from build123d import *

# Parameters (mm, degrees)
F0_W     = 101.6
F0_H     = 127
F1_DEPTH = 19.05
F2_W     = 76.2
F2_H     = 19.05
F3_DEPTH = 9.525
F4_R     = 6.35
F6_DEPTH = 19.051
F7_R     = 5.08
F8_W     = 25.4
F8_H     = 19.05
F9_DEPTH = 127.001


with BuildPart() as f1:
    # F0 (on Top) → F1 (new body)
    with BuildSketch(Plane.XY):
        with Locations((50.8, 63.5)):
            Rectangle(F0_W, F0_H)
    extrude(amount=F1_DEPTH)

    # F2 (on face) → F3 (cut)
    with BuildSketch(Plane.XY.offset(19.05)):
        with Locations((38.1, 63.5)):
            Rectangle(F2_W, F2_H)
    extrude(amount=-F3_DEPTH, mode=Mode.SUBTRACT)

    # F4
    f4_edges = [f1.edges().sort_by_distance(p)[0] for p in [
        (76.2, 73.025, 14.2875),
        (76.2, 53.975, 14.2875),
    ]]
    fillet(f4_edges, radius=F4_R)

    # F5 (on face) → F6 (cut, through all)
    with BuildSketch(Plane.XY.offset(19.05)):
        with BuildLine():
            ThreePointArc((25.4, 34.925), (22.225, 31.75), (25.4, 28.575))
            Line((25.4, 28.575), (76.2, 28.575))
            ThreePointArc((76.2, 28.575), (79.375, 31.75), (76.2, 34.925))
            Line((76.2, 34.925), (25.4, 34.925))
        make_face()
        with BuildLine():
            ThreePointArc((25.4, 98.425), (22.225, 95.25), (25.4, 92.075))
            Line((25.4, 92.075), (76.2, 92.075))
            ThreePointArc((76.2, 92.075), (79.375, 95.25), (76.2, 98.425))
            Line((76.2, 98.425), (25.4, 98.425))
        make_face()
    extrude(amount=-F6_DEPTH, mode=Mode.SUBTRACT)

    # F7
    f7_edges = [f1.edges().sort_by_distance(p)[0] for p in [
        (101.6, 0, 9.525),
        (101.6, 127, 9.525),
    ]]
    fillet(f7_edges, radius=F7_R)

    # F8 (on face) → F9 (cut, through all)
    with BuildSketch(Plane.XZ):
        with Locations((-3.175, 19.05)):
            Rectangle(F8_W, F8_H)
    extrude(amount=-F9_DEPTH, mode=Mode.SUBTRACT)


solid = f1.part
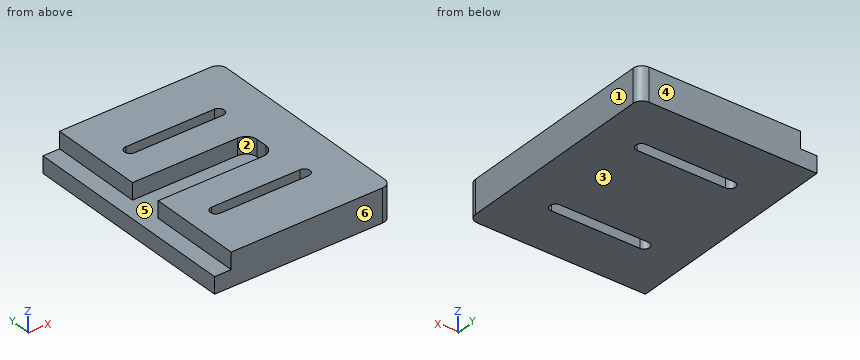
Verification items for the finished model (mm, model axes). Face numbers are marked on the shaded views. A direction names the side the tool comes from. Round coordinates to 2 decimals unless told otherwise and drop trailing zeros. Loops run counter-clockwise (first coordinate to the right, second up) from the corner with the lowest first, then second, coordinate; pieces in that order, holes last. Notation, with made-up numbers: M -26.5,63.25 L 13.5,63.25 A11 ccw 13.5,70.25 Z; hole C -5.75,0 d8. An arc over 180 degrees is marked long. Write each question's results on one line, items separated by ' | '.
1) Section check D-D on x = 15. Record the boundary of the cut face in (y, z) (3 decimals).
Checks:
outline: M 0,0 L 127,0 L 127,19.05 L 73.025,19.05 L 73.025,9.525 L 53.975,9.525 L 53.975,19.05 L 0,19.05 Z
2) Section check C-C on z = 16. Record the boundary of the cut face in (x, y) (3 decimals), then the cut area to 3 significant figures.
Checks:
outline: M 9.525,0 L 96.52,0 A5.08 ccw 101.6,5.08 L 101.6,121.92 A5.08 ccw 96.52,127 L 9.525,127 L 9.525,73.025 L 69.85,73.025 A6.35 cw 76.2,66.675 L 76.2,60.325 A6.35 cw 69.85,53.975 L 9.525,53.975 Z; hole M 25.4,28.575 L 76.2,28.575 A3.175 ccw 76.2,34.925 L 25.4,34.925 A3.175 ccw Z; hole M 25.4,92.075 L 76.2,92.075 A3.175 ccw 76.2,98.425 L 25.4,98.425 A3.175 ccw Z | area: 9,720 mm2
3) Section check B-B on x = 59. Record the boundary of the cut face in (y, z) (3 decimals).
Checks:
outline: M 0,0 L 28.575,0 L 28.575,19.05 L 0,19.05 Z; M 34.925,0 L 92.075,0 L 92.075,19.05 L 73.025,19.05 L 73.025,9.525 L 53.975,9.525 L 53.975,19.05 L 34.925,19.05 Z; M 98.425,0 L 127,0 L 127,19.05 L 98.425,19.05 Z
4) Section check A-A on y = 95.25. Record the boundary of the cut face in (x, z) (3 decimals).
Checks:
outline: M 0,0 L 22.225,0 L 22.225,19.05 L 9.525,19.05 L 9.525,9.525 L 0,9.525 Z; M 79.375,0 L 101.6,0 L 101.6,19.05 L 79.375,19.05 Z
5) Access from +Z, -Z, +X, -X, +Y, -Y to the whole of each face (thin tool, end or side, straight path). Record for the marked faces 1 and 2.
Checks:
face 1: +Z, -Z, +X, +Y, -Y | face 2: +Z, -X
6) Gauge pin test, flat ends, axial feed: P1, Ø3, axis at y = 63.5, z = 16, coming from the -X side; P2, Ø3, axis at y = 99, z = 12.5, coming from the -X side (3 decimals). Record the tip position at first contact, or that the pin passes through.
Checks:
P1: stops at x = 76.2 | P2: stops at x = 9.525
7) Scan lines: L1, parallel to Y at x = 33.5, z = 14.5 (3 decimals); L2, parallel to Y at x = 29, z = 1.25 (3 decimals); L3, parallel to Y at x = 24, z = 17.5 (3 decimals). Record each from-to range of solid material in increasing order. Write a range as from..to.
Checks:
L1: y = 0..28.575, 34.925..53.975, 73.025..92.075, 98.425..127 | L2: y = 0..28.575, 34.925..92.075, 98.425..127 | L3: y = 0..28.9, 34.6..53.975, 73.025..92.4, 98.1..127
8) Mould release check, pull along Y, two halves, no side actions. Record for the marked faces 3, 4, 5 and 6: released by +Y, released by -Y, zero draft, split by the parting line, or undercut.
Checks:
face 3: zero draft | face 4: released by +Y | face 5: undercut | face 6: released by -Y
